The listing builds one solid part. Answer for the finished solid, in the listing's coordinates (mm). A direction names the side the tool comes from. Coordinates: 2 decimals unless noted, no trailing zeros. Loops run counter-clockwise (first coordinate to the right, second up) from the corner with the lowest first, then second, coordinate; pieces in that order, holes last. Notation, with made-up numbers: (86.5, -30) - (105.5, -30) arc R19 cw to (105.5, -3) - close; hole circle Ø5 at (44, 48.5). An arc over 180 degrees is marked (long way). One line per question, with ' | ' between items.
Autodesk Inventor part; units mm, degrees
ref_plane "YZ Plane" through (0, 0, 0) normal (1, 0, 0) x (0, 1, 0)
ref_plane "XZ Plane" through (0, 0, 0) normal (0, 1, 0) x (-1, 0, 0)
ref_plane "XY Plane" through (0, 0, 0) normal (0, 0, 1) x (1, 0, 0)
sketch "Sketch20" plane through (0, 0, 0) normal (0, 1, 0) x (-1, 0, 0)
  line L0 (1.5185, -0.8925) -> (-3.5615, -0.8925)
  line L1 (-3.5615, -0.8925) -> (-3.5615, 11.8075)
  line L2 (-3.5615, 11.8075) -> (1.5185, 11.8075)
  line L3 (1.5185, 11.8075) -> (1.5185, -0.8925)
  line L4 (1.5185, 4.9634) -> (-3.5615, 4.9634)
  point P0 (0, 0)
  dimension "d56" = 5.08
  dimension "d57" = 12.7
extrude "Extrusion7" add sketch "Sketch20" along normal blind 2.54 contours L0 L1 L4 L3
extrude "Extrusion8" add sketch "Sketch20" along normal blind 6.35 contours L4 L1 L2 L3
sketch "Sketch21" plane through (0, 2.54, 0) normal (0, 1, 0) x (1, 0, 0)
  line L0 (3.5615, 0.8925) -> (-1.5185, 0.8925)
  line L1 (-1.5185, 0.8925) -> (-1.5185, -4.9634)
  point P0 (0, 0)
  point P1 (1.0215, -1.6475)
  dimension "d62" = 2.54
  dimension "d63" = 2.54
hole "Hole5" at (1.0215, 2.54, 1.6475) direction (0, -1, 0) diameter 2.4867 end through all
sketch "Sketch22" plane through (3.5615, 0, -0.8925) normal (1, 0, 0) x (0, 0, -1)
  line L0 (-12.7, 6.35) -> (-5.8558, 6.35)
  line L1 (-12.7, 0) -> (-12.7, 6.35)
  point P0 (-0.8925, 0)
  point P1 (-7.493, 3.175)
  dimension "d71" = 3.175
  dimension "d72" = 5.207
hole "Hole6" at (3.5615, 3.175, 6.6005) direction (-1, 0, 0) diameter 2.459 end through all
sketch "Sketch23" plane through (0, 2.54, 0) normal (0, 1, 0) x (1, 0, 0)
  line L0 (-1.5185, 0.8925) -> (-1.5185, -4.9634)
  line L1 (-1.5185, -4.9634) -> (-1.5185, -3.6934)
  line L2 (-1.5185, -3.6934) -> (3.5615, -3.6934)
  line L3 (3.5615, -4.9634) -> (3.5615, 0.8925)
  line L4 (3.5615, -3.6934) -> (3.5615, -4.9634)
  line L5 (3.5615, -11.8075) -> (3.5615, 0.8925)
  line L6 (3.5615, -4.9634) -> (-1.5185, -4.9634)
  line L7 (-1.5185, -4.9634) -> (3.5615, -4.9634)
  point P0 (0, 0)
  dimension "d80" = 1.27
extrude "Extrusion9" add sketch "Sketch23" along normal blind 3.81
properties part number "filament holders"
Item 1: Find section A-A, the plane x = 0.5. State how many separate pieces and enclosed holes the cut face has, plus the area to 3 significant figures.
Taken from the geometry:
separate pieces: 2 | enclosed holes: 1 | area: 52.7 mm2
Item 2: Find the intervals of material crossed by line 1 (Z direction, x = 0.35, y = 3.25); line 2 (Z direction, x = -0.2, y = 4.5); line 3 (Y direction, x = -0.05, z = 5.75), in increasing order. Write a range as [from, to].
Taken from the geometry:
line 1: z = [3.69, 5.37], [7.83, 11.81] | line 2: z = [3.69, 11.81] | line 3: y = [0, 2.29], [4.06, 6.35]
Item 3: The mould has two halves that part along X. Classify faces 1 (the face through (3.562, 1.7, 7)), 2 (the face through (0.648, 1.252, 2.833)), 3 (the face through (1, 6.35, 8)): pulls with the +X half, pulls with the -X half, needs draft (parallel to the pull), parting line crosses it, or undercut.
Taken from the geometry:
face 1: pulls with the +X half | face 2: undercut | face 3: needs draft
Item 4: Each of these flat-tipped pins is pushed along its axis until it touches: pin 1 Ø3 at (x, y) = (1, 3.5) entering from -Z; pin 2 Ø2 at (y, z) = (3.18, 6.6) entering from -X; pin 3 Ø1.9 at (x, y) = (0.5, 4) entering from -Z. Where does it stop, or does it pass through?
Taken from the geometry:
pin 1: stops at z = -0.89 | pin 2: passes through | pin 3: stops at z = 3.69
Item 5: Find section D-D, the plane y = 0.5. Write down the section's boundary in (x, z), plus the area to 3 significant figures.
Taken from the geometry:
outline: (-1.52, -0.89) - (3.56, -0.89) - (3.56, 11.81) - (-1.52, 11.81) - close; hole circle Ø2.49 at (1.02, 1.65) | area: 59.7 mm2
Item 6: Find section C-C, the plane z = 6.25. Write down the section's boundary in (x, y).
Taken from the geometry:
outline: (-1.52, 0) - (3.56, 0) - (3.56, 2) - (-1.52, 2) - close; (-1.52, 4.35) - (3.56, 4.35) - (3.56, 6.35) - (-1.52, 6.35) - close
Item 7: Find section B-B, the plane y = 2.75. Write down the section's boundary in (x, z).
Taken from the geometry:
outline: (-1.52, 3.69) - (3.56, 3.69) - (3.56, 5.45) - (-1.52, 5.45) - close; (-1.52, 7.75) - (3.56, 7.75) - (3.56, 11.81) - (-1.52, 11.81) - close
Item 8: Which of the six approach directions +Z, -Z, +X, -X, +Y, -Y give full straight-line access (tool end or side, diameter ignored) to faces 4 (the face through (1, 0, 6)), 5 (the face through (0, 2.54, 0))?
Taken from the geometry:
face 4: +Z, -Z, +X, -X, -Y | face 5: -Z, +X, -X, +Y
